Autodesk Inventor part; units mm, degrees
ref_plane "Start Plane" through (0, 0, -14.2929) normal (0, 0, 1) x (1, 0, 0)
ref_plane "End Plane" through (0, 0, 1414.2929) normal (0, 0, 1) x (1, 0, 0)
ref_plane "Work Plane11" through (-7.7636, 7.7, -14.6464) normal (0.7071, 0, -0.7071) x (-0.7071, 0, -0.7071)
ref_plane "Start Plane" through (0, 0, -14.2929) normal (0, 0, 1) x (1, 0, 0)
ref_plane "End Plane" through (0, 0, 1414.2929) normal (0, 0, 1) x (1, 0, 0)
sketch "Sketch" plane through (0, 0, 0) normal (0, 0, 1) x (1, 0, 0)
  line L0 (-2.41, 28.7) -> (-2.41, -7.3)
  line L1 (-7.41, 32.7) -> (-6.41, 32.7)
  line L2 (-7.41, -17.3) -> (-7.41, 32.7)
  line L3 (22.59, -17.3) -> (-7.41, -17.3)
  line L4 (22.59, -16.3) -> (22.59, -17.3)
  line L5 (2.59, -12.3) -> (18.59, -12.3)
  arc A0 (-2.41, -7.3) -> (2.59, -12.3) centre (2.59, -7.3) ccw
  arc A1 (-2.41, 28.7) -> (-6.41, 32.7) centre (-6.41, 28.7) ccw
  arc A2 (22.59, -16.3) -> (18.59, -12.3) centre (18.59, -16.3) ccw
  line L6 (0, 43.6941) -> (0, -27.4657) construction
  line L7 (-13.5757, 0) -> (29.5841, 0) construction
  point P0 (-2.41, 32.7)
  point P1 (-2.41, -12.3)
  point P2 (22.59, -12.3)
  dimension "d4" = 30
  dimension "d6" = 50
  dimension "d8" = 5
  dimension "d10" = 5
  dimension "d17" = 5
  dimension "d18" = 4
  dimension "d19" = 17.3
  dimension "d20" = 7.41
extrude "Body" add sketch "Sketch" along normal up to surface (1428.5858 mm away) from surface at -14.2929
sketch "Sketch3" plane through (0, 0, 0) normal (0, 0, 1) x (1, 0, 0)
  line L0 (0, 0) -> (10, 0)
ref_plane "Work Plane10" through (0, 0, 0) normal (0, -1, 0) x (1, 0, 0)
sketch "Sketch4" plane through (0, 0, 0) normal (0, -1, 0) x (1, 0, 0)
  line L0 (-2, -14.2929) -> (12, -14.2929)
  line L1 (-2, 1414.2929) -> (12, 1414.2929)
  dimension "d24" = 1428.5858
ref_plane "Work Plane11" through (-7.7636, 7.7, -14.6464) normal (0.7071, 0, -0.7071) x (-0.7071, 0, -0.7071)
split "Split1" plane through (-7.7636, 7.7, -14.6464) removes the side toward (0.7071, 0, -0.7071)
ref_plane "Work Plane12" through (-7.7636, 7.7, 1414.6464) normal (0.7071, 0, 0.7071) x (0.7071, 0, -0.7071)
split "Split2" plane through (-7.7636, 7.7, 1414.6464) removes the side toward (0.7071, 0, 0.7071)
equation "\"d4\" = b"
equation "\"d6\" = ParH"
equation "\"d17\" = R"
equation "\"d18\" = R1"
equation "\"d19\" = ex"
equation "\"d20\" = ey"
equation "\"d11\" = G_L"
equation "\"b\" = 30"
equation "\"ParT\" = 5"
equation "\"R1\" = 4"
equation "\"G_L\" = d24"
equation "\"ParH\" = 50"
equation "\"R\" = 5"
equation "\"ey\" = 7.41"
equation "\"ex\" = 17.3"
equation "\"G_OFFSET_START\" = 14.29289"
equation "\"G_OFFSET_END\" = 14.29289"
equation "\"d21\" = -G_OFFSET_START"
equation "\"d22\" = G_OFFSET_END + B_L"
properties part number "ISO 657-2 - 50x 30x 5-1428.59" material "Steel, Mild"
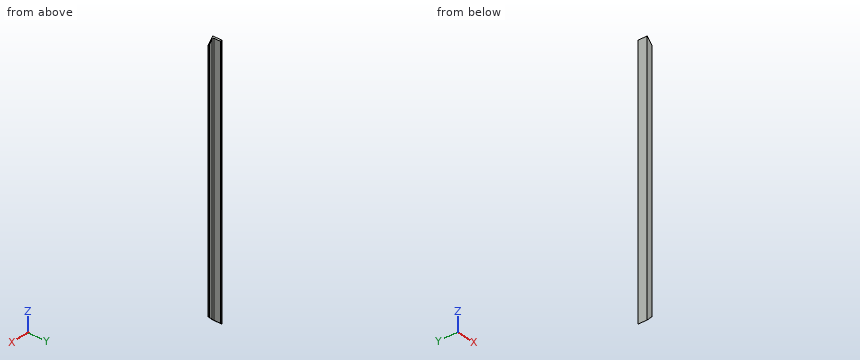
Geometry check sheet. Reference: the model listing, model coordinates, mm. Round coordinates to 2 decimals unless told otherwise and drop trailing zeros. Loops run counter-clockwise (first coordinate to the right, second up) from the corner with the lowest first, then second, coordinate; pieces in that order, holes last.
Item 1: Cross-section at B-B on y = 6.5. Record the boundary of the cut face in (x, z).
Item 2: Thickness scan on line 1 (Y direction, x = 9, z = 94); line 2 (X direction, y = 4, z = 1092); line 3 (Y direction, x = -5, z = 362). Record the ranges inside material, lowest first.
Item 3: Cross-section at A-A on z = 517.5. Record the boundary of the cut face in (x, y), then the cut area to 3 significant figures.
Item 4: Gauge pin test, flat ends, axial feed: pin 1 (5 mm diameter, centred on y = -3.5, z = 260, fed in from +X); pin 2 (5 mm diameter, centred on x = 12, z = 786.5, fed in from +Y); pin 3 (5 mm diameter, centred on x = -4, y = 4.5, fed in from -Z). Record the tip position at first contact, or that the pin passes through.
Item 5: Cross-section at C-C on x = 7.5. Record the boundary of the cut face in (y, z).
Answer sheet:
1. outline: (-7.41, -14.29) - (-2.41, -9.29) - (-2.41, 1409.29) - (-7.41, 1414.29) - close
2. line 1: y = -17.3 to -12.3
2. line 2: x = -7.41 to -2.41
2. line 3: y = -17.3 to 32.44
3. outline: (-7.41, -17.3) - (22.59, -17.3) - (22.59, -16.3) arc R4 ccw to (18.59, -12.3) - (2.59, -12.3) arc R5 cw to (-2.41, -7.3) - (-2.41, 28.7) arc R4 ccw to (-6.41, 32.7) - (-7.41, 32.7) - close
3. area: 373 mm2
4. pin 1: stops at x = -2.41
4. pin 2: stops at y = -12.3
4. pin 3: stops at z = -13.38
5. outline: (-17.3, 0.62) - (-12.3, 0.62) - (-12.3, 1399.38) - (-17.3, 1399.38) - close
